Design review of the part built by this model. Coordinates are the model's own, in mm. A direction names the side the tool comes from. Round coordinates to 2 decimals unless told otherwise and drop trailing zeros. Write each loop counter-clockwise with the first axis right and the second up, starting at its lowest first coordinate (ties: lowest second). Pieces come first, ordered by that corner, then holes. Notation, with made-up numbers: (-13, -10) -> (10, -10) arc R11 cw to (10, -6) -> close; hole circle Ø9 at (46, 52.25). An arc over 180 degrees is marked (long way). Write item = value, one per line. Start each with the question number.
Item 1: Mouldability with a two-part tool opening along X and no side actions: class faces 1 (the flat face through (55.62, 15.21, -246.84)), 2 (the flat face through (-50.349, 17.325, 249.224)), 3 (the flat face through (0, 30, 289)) as released by +X, released by -X, zero draft, split by the parting line, or undercut.
Item 2: Add section B-B, the plane z = -189. State the section outline as (x, y) points, then the cut area to 3 significant figures.
Item 3: For pin 1 Ø12 at (x, y) = (87.5, 19.5) entering from -Z; pin 2 Ø7.5 at (x, y) = (87.5, 22.5) entering from -Z; pin 3 Ø1.5 at (y, z) = (18, -77.5) entering from +X; pin 4 Ø5 at (x, z) = (-6, -93.5) entering from -Y, all flat-tipped, find the tip position at first contact; note any pin that passes through.
Item 4: Add section A-A, the plane y = 10. State the section outline as (x, z) points.
Item 5: To check wall thickness, follow L1, parallel to Z at x = -29.5, y = 9.5; L2, parallel to Y at x = 32, z = -195.5; L3, parallel to X at y = 20, z = 73. State the ranges of each line that lie inside material, in increasing order.
Item 6: Add section D-D, the plane x = -32. State the section outline as (y, z) points, then the cut area to 3 significant figures.
Item 7: Machinability: for faces 4 (the flat face through (-84, 24, 15.25)), 5 (the flat face through (74.8, 17.3, -3.1)), 6 (the flat face through (84, 24, 105.25)), which of the approach directions +Z, -Z, +X, -X, +Y, -Y give a long, thin tool a straight path to every point of the face, cutting with its end or side? Answer none if there is none.
Item 8: Add section C-C, the plane x = -69.5. State the section outline as (y, z) points, then the cut area to 3 significant figures.
from build123d import *

# Parameters (mm, degrees)
BOSS_EXTRUDE1_DEPTH     = 5
BOSS_EXTRUDE2_DEPTH     = 224.75
BOSS_EXTRUDE3_DEPTH     = 25
SKETCH7_W               = 5
SKETCH7_H               = 5
BOSS_EXTRUDE5_DEPTH     = 15
BOSS_EXTRUDE6_DEPTH     = 50
BOSS_EXTRUDE7_DEPTH     = 48
BOSS_EXTRUDE8_DEPTH     = 48
BOSS_EXTRUDE9_DEPTH     = 48
CUT_EXTRUDE1_DEPTH      = 95.104275362
CUT_EXTRUDE1_DEPTH_BACK = 93.6900618
SKETCH20_W              = 50
SKETCH20_H              = 48.112885627
CUT_EXTRUDE2_DEPTH      = 105
CUT_EXTRUDE3_DEPTH      = 105
BOSS_EXTRUDE11_DEPTH    = 5
CUT_EXTRUDE4_DEPTH      = 293.4400618
CUT_EXTRUDE4_DEPTH_BACK = 278.247872606
CUT_EXTRUDE5_DEPTH      = 29
SKETCH25_W              = 15
SKETCH25_H              = 10
CUT_EXTRUDE6_DEPTH      = 26
CUT_EXTRUDE6_DEPTH_BACK = 6


with BuildPart() as part:
    # Sketch1 → Boss-Extrude1 (new body)
    with BuildSketch(Plane(origin=(0, 0, 0), x_dir=(1, 0, 0), z_dir=(0, 1, 0))):
        Polygon((62.497872606, -224.75), (62.497872606, 224.75), (25, 262.247872606), (-25, 262.247872606), (-62.497872606, 224.75), (-62.497872606, -224.75), (-25, -262.247872606), (25, -262.247872606), align=None)
    extrude(amount=BOSS_EXTRUDE1_DEPTH)

    # Sketch3 → Boss-Extrude2 (add, symmetric)
    with BuildSketch(Plane(origin=(0, 0, 0), x_dir=(0, -1, 0), z_dir=(0, 0, 1))):
        Polygon((0, 62.497872606), (-5, 62.497872606), (-30, 87.497872606), (-30, 92.497872606), align=None)
        Polygon((-30, -87.497872606), (-30, -92.497872606), (0, -62.497872606), (-5, -62.497872606), align=None)
    extrude(amount=BOSS_EXTRUDE2_DEPTH, both=True)

    # Sketch6 → Boss-Extrude3 (add, symmetric)
    with BuildSketch(Plane(origin=(0, 0, 0), x_dir=(0, -1, 0), z_dir=(-1, 0, 0))):
        Polygon((0, 262.247872606), (-30, 292.247872606), (-30, 287.247872606), (-5, 262.247872606), align=None)
        Polygon((0, -262.247872606), (-15, -277.247872606), (-15, -272.247872606), (-5, -262.247872606), align=None)
    extrude(amount=BOSS_EXTRUDE3_DEPTH, both=True)

    # Sketch7 → Boss-Extrude5 (add)
    with BuildSketch(Plane(origin=(0, 15, 0), x_dir=(1, 0, 0), z_dir=(0, 1, 0))):
        with Locations((-22.5, 274.747872606)):
            Rectangle(SKETCH7_W, SKETCH7_H)
        with Locations((22.5, 274.747872606)):
            Rectangle(SKETCH7_W, SKETCH7_H)
    extrude(amount=BOSS_EXTRUDE5_DEPTH)

    # Sketch10 → Boss-Extrude6 (add, symmetric)
    with BuildSketch(Plane(origin=(99.875, 0, -99.875), x_dir=(0, -1, 0), z_dir=(0.707106781, 0, -0.707106781))):
        Polygon((0, 203.114918601), (-30, 224.328122037), (-30, 220.792588131), (-5, 203.114918601), align=None)
    extrude(amount=BOSS_EXTRUDE6_DEPTH, both=True)

    # Sketch13 → Boss-Extrude7 (add, symmetric)
    with BuildSketch(Plane(origin=(-99.875, 0, -99.875), x_dir=(0, -1, 0), z_dir=(0.707106781, 0, 0.707106781))):
        Polygon((-5, 203.114918601), (-30, 220.792588131), (-30, 224.328122037), (0, 203.114918601), align=None)
    extrude(amount=BOSS_EXTRUDE7_DEPTH, both=True)

    # Sketch15 → Boss-Extrude8 (add, symmetric)
    with BuildSketch(Plane(origin=(-99.875, 0, 99.875), x_dir=(0, -1, 0), z_dir=(-0.707106781, 0, 0.707106781))):
        Polygon((-5, 203.114918601), (-30, 220.792588131), (-30, 224.328122037), (0, 203.114918601), align=None)
    extrude(amount=BOSS_EXTRUDE8_DEPTH, both=True)

    # Sketch17 → Boss-Extrude9 (add, symmetric)
    with BuildSketch(Plane(origin=(99.875, 0, 99.875), x_dir=(0, -1, 0), z_dir=(-0.707106781, 0, -0.707106781))):
        Polygon((-5, 203.114918601), (-30, 220.792588131), (-30, 224.328122037), (0, 203.114918601), align=None)
    extrude(amount=BOSS_EXTRUDE9_DEPTH, both=True)

    # Sketch18 → Cut-Extrude1 (cut, two sides)
    with BuildSketch(Plane(origin=(0, 0, 0), x_dir=(0, -1, 0), z_dir=(-1, 0, 0))) as cut_extrude1_sk:
        Polygon((0, 262.247872606), (-30, 292.4400618), (0, 277.4400618), align=None)
    extrude(amount=CUT_EXTRUDE1_DEPTH, mode=Mode.SUBTRACT)
    extrude(cut_extrude1_sk.sketch, amount=-CUT_EXTRUDE1_DEPTH_BACK, mode=Mode.SUBTRACT)

    # Sketch20 → Cut-Extrude2 (cut)
    with BuildSketch(Plane(origin=(0, -131.123936303, -131.123936303), x_dir=(1, 0, 0), z_dir=(0, -0.707106781, -0.707106781))):
        with Locations((0, -209.493691886)):
            Rectangle(SKETCH20_W, SKETCH20_H)
    extrude(amount=CUT_EXTRUDE2_DEPTH, mode=Mode.SUBTRACT)

    # Sketch21 → Cut-Extrude3 (cut)
    with BuildSketch(Plane(origin=(0, 0, -277.247872606), x_dir=(-1, 0, 0), z_dir=(0, 0, -1))):
        Polygon((20, 15), (-53.678843976, 15), (-53.678843976, 30), (47.571265033, 30), (47.571265033, 15), align=None)
    extrude(amount=CUT_EXTRUDE3_DEPTH, mode=Mode.SUBTRACT)

    # Sketch22 → Boss-Extrude11 (add)
    with BuildSketch(Plane(origin=(0, 0, -277.247872606), x_dir=(-1, 0, 0), z_dir=(0, 0, -1))):
        Polygon((-40, 30), (-25, 15), (-20, 15), (-20, 30), align=None)
        Polygon((20, 30), (40, 30), (25, 15), (20, 15), align=None)
    extrude(amount=-BOSS_EXTRUDE11_DEPTH)

    # Sketch23 → Cut-Extrude4 (cut, two sides)
    with BuildSketch(Plane(origin=(0, 0, 0), x_dir=(0, -1, 0), z_dir=(0, 0, 1))) as cut_extrude4_sk:
        Polygon((0, 62.497872606), (-30, 92.6900618), (0, 77.6900618), align=None)
    extrude(amount=CUT_EXTRUDE4_DEPTH, mode=Mode.SUBTRACT)
    extrude(cut_extrude4_sk.sketch, amount=-CUT_EXTRUDE4_DEPTH_BACK, mode=Mode.SUBTRACT)

    # Sketch24 → Cut-Extrude5 (cut)
    with BuildSketch(Plane(origin=(-31.248936303, -31.248936303, 0), x_dir=(0, 0, 1), z_dir=(-0.707106781, -0.707106781, 0))):
        Polygon((-224.75, 44.19266953), (-259.614343039, 44.19266953), (-259.614343039, 90.205869936), (275.937456007, 90.205869936), (275.937456007, 44.19266953), align=None)
    extrude(amount=CUT_EXTRUDE5_DEPTH, mode=Mode.SUBTRACT)

    # Sketch25 → Cut-Extrude6 (cut, two sides)
    with BuildSketch(Plane(origin=(0, 5, 0), x_dir=(1, 0, 0), z_dir=(0, 1, 0))) as cut_extrude6_sk:
        with Locations((84.997872606, 214.75)):
            Rectangle(SKETCH25_W, SKETCH25_H)
        with Locations((84.997872606, 169.75)):
            Rectangle(SKETCH25_W, SKETCH25_H)
        with Locations((84.997872606, 124.75)):
            Rectangle(SKETCH25_W, SKETCH25_H)
        with Locations((84.997872606, 79.75)):
            Rectangle(SKETCH25_W, SKETCH25_H)
        with Locations((84.997872606, 34.75)):
            Rectangle(SKETCH25_W, SKETCH25_H)
        with Locations((84.997872606, -10.25)):
            Rectangle(SKETCH25_W, SKETCH25_H)
        with Locations((84.997872606, -55.25)):
            Rectangle(SKETCH25_W, SKETCH25_H)
        with Locations((84.997872606, -190.25)):
            Rectangle(SKETCH25_W, SKETCH25_H)
        with Locations((84.997872606, -145.25)):
            Rectangle(SKETCH25_W, SKETCH25_H)
        with Locations((84.997872606, -100.25)):
            Rectangle(SKETCH25_W, SKETCH25_H)
        with Locations((-84.997872606, -190.25)):
            Rectangle(SKETCH25_W, SKETCH25_H)
        with Locations((-84.997872606, -145.25)):
            Rectangle(SKETCH25_W, SKETCH25_H)
        with Locations((-84.997872606, -100.25)):
            Rectangle(SKETCH25_W, SKETCH25_H)
        with Locations((-84.997872606, -55.25)):
            Rectangle(SKETCH25_W, SKETCH25_H)
        with Locations((-84.997872606, 34.75)):
            Rectangle(SKETCH25_W, SKETCH25_H)
        with Locations((-84.997872606, 214.75)):
            Rectangle(SKETCH25_W, SKETCH25_H)
        with Locations((-84.997872606, 169.75)):
            Rectangle(SKETCH25_W, SKETCH25_H)
        with Locations((-84.997872606, 124.75)):
            Rectangle(SKETCH25_W, SKETCH25_H)
        with Locations((-84.997872606, 79.75)):
            Rectangle(SKETCH25_W, SKETCH25_H)
        with Locations((-84.997872606, -10.25)):
            Rectangle(SKETCH25_W, SKETCH25_H)
    extrude(amount=CUT_EXTRUDE6_DEPTH, mode=Mode.SUBTRACT)
    extrude(cut_extrude6_sk.sketch, amount=-CUT_EXTRUDE6_DEPTH_BACK, mode=Mode.SUBTRACT)


solid = part.part
Result set:
q1.face_1 = released by +X
q1.face_2 = undercut
q1.face_3 = zero draft
q2.outline = (-92.5, 30) -> (-62.5, 0) -> (62.5, 0) -> (92.5, 30) -> (87.5, 30) -> (62.5, 5) -> (-62.5, 5) -> (-87.5, 30) -> close
q2.area = 900 mm²
q3.pin_1 = -227.73
q3.pin_2 = -227.55
q3.pin_3 = 77.5
q3.pin_4 = 0
q4.outline = (-72.5, -224.75) -> (-25, -272.25) -> (25, -272.25) -> (72.56, -224.69) -> (72.56, -219.69) -> (72.5, -219.75) -> (72.5, 219.75) -> (72.56, 219.69) -> (72.56, 224.69) -> (24.94, 272.31) -> (19.94, 272.31) -> (20, 272.25) -> (-20, 272.25) -> (-19.94, 272.31) -> (-24.94, 272.31) -> (-72.5, 224.75) -> close; hole (-67.5, -224.75) -> (-25, -267.25) -> (25, -267.25) -> (67.5, -224.75) -> (67.5, 224.75) -> (25, 267.25) -> (-25, 267.25) -> (-67.5, 224.75) -> close
q5.L1 = -267.25 to -262.25, 262.25 to 267.25
q5.L2 = 0 to 5
q5.L3 = -82.5 to -77.5, 77.5 to 82.5
q6.outline = (0, -255.25) -> (22, -277.25) -> (30, -277.25) -> (30, -272.25) -> (22, -272.25) -> (5, -255.25) -> (5, 255.25) -> (30, 280.25) -> (30, 285.25) -> (0, 255.25) -> close
q6.area = 2,830 mm²
q7.face_4 = -X, +Y, -Y
q7.face_5 = +Y
q7.face_6 = +X, +Y, -Y
q8.outline = (7, -224.75) -> (30, -247.75) -> (30, -242.75) -> (12, -224.75) -> (12, 224.75) -> (30, 242.75) -> (30, 247.75) -> (7, 224.75) -> close
q8.area = 2,450 mm²
